from build123d import *

# Parameters (mm, degrees)
F0_W     = 40
F0_H     = 30
F1_DEPTH = 5
F2_R     = 8
F3_DEPTH = 25
F4_W     = 35
F4_H     = 5
F5_DEPTH = 30
F6_W     = 35
F6_H     = 5
F7_DEPTH = 10


with BuildPart() as f1:
    # F0 (on Front) → F1 (new body)
    with BuildSketch(Plane.XZ):
        Rectangle(F0_W, F0_H)
    extrude(amount=F1_DEPTH)

    # F2 (on face) → F3 (cut)
    with BuildSketch(Plane.XZ.offset(5)):
        Circle(F2_R)
    extrude(amount=-F3_DEPTH, mode=Mode.SUBTRACT)

    # F4 (on face) → F5 (join)
    with BuildSketch(Plane.XZ.offset(5)):
        Polygon((15, -15), (20, -15), (20, 15), (15, 15), (15, 10), align=None)
        with Locations((-2.5, 12.5)):
            Rectangle(F4_W, F4_H)
    extrude(amount=F5_DEPTH)

    # F6 (on face) → F7 (join)
    with BuildSketch(Plane.XZ.offset(5)):
        with Locations((-2.5, -12.5)):
            Rectangle(F6_W, F6_H)
    extrude(amount=F7_DEPTH)


solid = f1.part
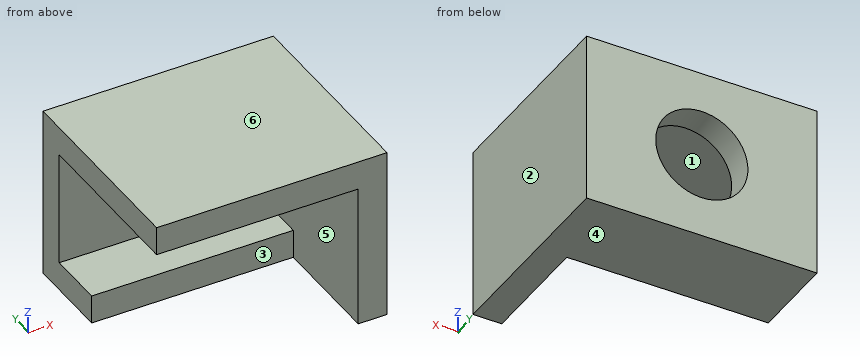
The model under review builds one solid part; all positions refer to its coordinate system, in mm. Face numbers are marked on the shaded views. A direction names the side the tool comes from. Give positions to 0.01 mm unless a question says otherwise; leave off trailing zeros. Loops run counter-clockwise (first coordinate to the right, second up) from the corner with the lowest first, then second, coordinate; pieces in that order, holes last. Notation, with made-up numbers: (25.5, 31.25) -> (64.5, 31.25) arc R29 ccw to (64.5, 56.25) -> close; hole circle Ø2 at (57, -1.5). An arc over 180 degrees is marked (long way). Put each result on its own line as item: value. Start each with the question number.
1. For the marked faces 1, 2 and 3, list the 3-axis set-ups (+Z, -Z, +X, -X, +Y, -Y) from which the entire face can be reached by the end or side of a thin tool; tool diameter is ignored.
2. We need section B-B on y = -4. State the section outline as (x, z) points, then the cut area to 3 significant figures.
3. Clearance check with flat-ended pins moving along their axes: P1, Ø5, axis at y = -8.5, z = -4.5, coming from the -X side; P2, Ø1.5, axis at x = 2.5, z = 9, coming from the -Y side; P3, Ø10, axis at x = -6, y = -18.5, coming from the -Z side; P4, Ø8, axis at x = 2, z = 1.5, coming from the -Y side. State where each tip first meets the part, or that it passes through.
4. Wall thickness on probe 1 along Z at (x, y) = (0, -1.35); probe 2 along Z at (x, y) = (11.5, -14.5); probe 3 along Y at (x, z) = (-16, 4.5): over which ranges is each line inside the solid? List them lowest first.
5. We need section A-A on x = 0. State the section outline as (y, z) points, then the cut area to 3 significant figures.
6. We need section C-C on z = 0. State the section outline as (x, y) points, then the cut area to 3 significant figures.
7. We need section D-D on y = -16. State the section outline as (x, z) points, then the cut area to 3 significant figures.
8. Mouldability with a two-part tool opening along Z and no side actions: class the marked faces 4, 5 and 6 as released by +Z, released by -Z, zero draft, split by the parting line, or undercut.
Determined:
1. face 1: -X, -Y
1. face 2: +Z, -Z, +X, +Y, -Y
1. face 3: -Z, -X, -Y
2. outline: (-20, -15) -> (20, -15) -> (20, 15) -> (-20, 15) -> close; hole circle Ø16 at (0, 0)
2. area: 999 mm^2
3. P1: x = 15
3. P2: y = -5
3. P3: z = -15
3. P4: through
4. probe 1: -15 to -8, 8 to 15
4. probe 2: -15 to -10, 10 to 15
4. probe 3: -5 to 0
5. outline: (-35, 10) -> (-5, 10) -> (-5, 8) -> (0, 8) -> (0, 15) -> (-35, 15) -> close; (-15, -15) -> (0, -15) -> (0, -8) -> (-5, -8) -> (-5, -10) -> (-15, -10) -> close
5. area: 270 mm^2
6. outline: (-20, -5) -> (-8, -5) -> (-8, 0) -> (-20, 0) -> close; (8, -5) -> (15, -5) -> (15, -35) -> (20, -35) -> (20, 0) -> (8, 0) -> close
6. area: 270 mm^2
7. outline: (-20, 10) -> (15, 10) -> (15, -15) -> (20, -15) -> (20, 15) -> (-20, 15) -> close
7. area: 325 mm^2
8. face 4: released by -Z
8. face 5: undercut
8. face 6: released by +Z
